CAD build for the part. Positions are in the model's coordinates, mm. Face numbers are marked on the shaded views. A direction names the side the tool comes from. Give positions to 0.01 mm unless a question says otherwise; leave off trailing zeros. Write each loop counter-clockwise with the first axis right and the second up, starting at its lowest first coordinate (ties: lowest second). Pieces come first, ordered by that corner, then holes. Notation, with made-up numbers: (-40, 5) - (-11, 5) arc R14 ccw to (-11, 21) - close; hole circle Ø7 at (32.25, -4). An arc over 180 degrees is marked (long way). Answer as a JSON object with one key per item and string values.
Solid Edge part; units mm, degrees
sketch "Sketch1" plane through (0, 0, 0) normal (0, -1, 0) x (1, 0, 0)
  line L0 (-8.05, -17.5) -> (8.05, -17.5)
  line L1 (8.05, -17.5) -> (8.05, 17.5)
  line L2 (8.05, 17.5) -> (-8.05, 17.5)
  line L3 (-8.05, 17.5) -> (-8.05, -17.5)
  dimension "D1" = 8.05
  dimension "D2" = 8.05
extrude "Protrusion1" add sketch "Sketch1" against normal blind 2
sketch "Sketch2" plane through (0, 0, 0) normal (0, -1, 0) x (1, 0, 0)
  line L0 (-10.05, -19.5) -> (10.05, -19.5)
  line L1 (10.05, -19.5) -> (10.05, 19.5)
  line L2 (10.05, 19.5) -> (-10.05, 19.5)
  line L3 (-10.05, 19.5) -> (-10.05, -19.5)
  line L4 (-8.05, -17.5) -> (8.05, -17.5)
  line L5 (8.05, -17.5) -> (8.05, 17.5)
  line L6 (8.05, 17.5) -> (-8.05, 17.5)
  line L7 (-8.05, 17.5) -> (-8.05, -17.5)
extrude "Extrusionsausprägung_2" add sketch "Sketch2" against normal blind 9
sketch "Sketch3" plane through (0, 0, 0) normal (0, -1, 0) x (1, 0, 0)
  circle A0 centre (0, 9.5) radius 5
extrude "Cutout1" cut sketch "Sketch3" against normal through all
sketch "Sketch4" plane through (0, 0, 0) normal (0, -1, 0) x (1, 0, 0)
  line L0 (-4.75, 7.9388) -> (4.75, 7.9388)
  line L1 (4.75, 7.9388) -> (4.75, -0.0612)
  line L2 (4.75, -0.0612) -> (-4.75, -0.0612)
  line L3 (-4.75, -0.0612) -> (-4.75, 7.9388)
  dimension "D1" = 4.75
  dimension "D2" = 4.75
extrude "Cutout2" cut sketch "Sketch4" against normal through all
chamfer "Fase_1" distance 0.5 angle 45 8 edges at (0, 9, 19.5) (0, 9, 17.5) (10.05, 9, 0) (8.05, 9, 0) (-8.05, 9, 0) (-10.05, 9, 0) (0, 9, -19.5) (0, 9, -17.5)
sketch "Sketch5" plane through (10.05, 5.75, 0) normal (1, 0, 0) x (0, 0, -1)
  line L0 (-19.5, -3.75) -> (-9.5, -3.75)
  line L1 (-9.5, -3.75) -> (-9.5, 3.25)
  line L2 (-9.5, 3.25) -> (-19.5, 3.25)
  line L3 (-19.5, 3.25) -> (-19.5, -3.75)
  line L4 (19.5, -3.75) -> (4.5, -3.75)
  line L5 (4.5, -3.75) -> (4.5, 3.25)
  line L6 (4.5, 3.25) -> (19.5, 3.25)
  line L7 (19.5, 3.25) -> (19.5, -3.75)
  dimension "D1" = 9.5
extrude "Cutout3" cut sketch "Sketch5" against normal through all
chamfer "Fase_3" distance 0.5 angle 45 8 edges at (10.05, 5.25, -4.5) (8.05, 5.25, -4.5) (-8.05, 5.25, -4.5) (-10.05, 5.25, -4.5) (-8.05, 5.25, 9.5) (-10.05, 5.25, 9.5) (8.05, 5.25, 9.5) (10.05, 5.25, 9.5)
sketch "Sketch6" plane through (0, 2, 0) normal (0, 1, 0) x (-1, 0, 0)
  line L0 (-10.05, 19.5) -> (10.05, 19.5)
  line L1 (10.05, 19.5) -> (10.05, 16.5)
  line L2 (10.05, 16.5) -> (-10.05, 16.5)
  line L3 (-10.05, 16.5) -> (-10.05, 19.5)
  dimension "D1" = 10.05
extrude "Cutout4" cut sketch "Sketch6" against normal through all
fillet "Verrundung_4" radius 7 2 edges at (10.05, 1, 16.5) (-10.05, 1, 16.5)
sketch "Sketch7" plane through (10.05, 4.25, -5) normal (1, 0, 0) x (0, -1, 0)
  line L0 (2.25, 14.5) -> (4.25, 14.5)
  line L1 (4.25, 14.5) -> (4.25, 3.5)
  line L2 (4.25, 3.5) -> (2.25, 3.5)
  line L3 (2.25, 3.5) -> (2.25, 14.5)
extrude "Cutout5" cut sketch "Sketch7" against normal through all
sketch "Sketch8" plane through (10.05, 4.25, 0.5) normal (1, 0, 0) x (0, -1, 0)
  arc A0 (2.25, 9) -> (-7.75, 19) centre (-7.75, 9) ccw
  line L0 (-7.75, 19) -> (-7.75, 21)
  arc A1 (-7.75, 21) -> (4.25, 9) centre (-7.75, 9) cw
  line L1 (4.25, 9) -> (2.25, 9)
extrude "Protrusion2" add sketch "Sketch8" against normal up to vertex (20.1 mm away)
fillet "Verrundung_5" radius 5 2 edges at (10.05, 12, -19.5) (-10.05, 12, -19.5)
fillet "Verrundung_6" radius 1.5 10 edges at (10.05, 1.9005, -14.9807) (10.05, 0, 0.5) (7.9997, 0, 14.4497) (0, 0, 16.5) (-7.9997, 0, 14.4497) (-10.05, 0, 0.5) (-10.05, 1.9005, -14.9807) (-8.6361, 10.4842, -20.4039) (0, 12, -20.5) (8.6361, 10.4842, -20.4039)
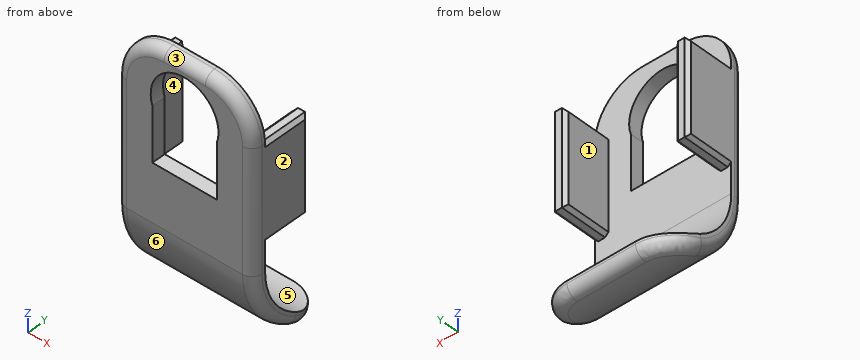
(1) Flat gauge pins, fed straight in: P1, Ø11.5, axis at x = 0, z = 9.5, coming from the +Y side; P2, Ø0.5, axis at x = 9, y = 5.5, coming from the +Z side; P3, Ø3, axis at x = -7, y = 1.5, coming from the +Z side. Where does each tip first touch, or does it go through?
Answer key:
{"P1": "stops at y = 2", "P2": "stops at z = 9.5", "P3": "stops at z = 16.06"}
(2) Saw through at A-A, the plane z = 7.5. Give the cut face in (x, y), and give its area (3 significant figures).
Answer key:
{"outline": "(-10.05, 1.5) arc R1.5 ccw to (-8.55, 0) - (-4.75, 0) - (-4.75, 2) - (-8.05, 2) - (-8.05, 8.5) - (-8.55, 9) - (-9.55, 9) - (-10.05, 8.5) - close; (4.75, 0) - (8.55, 0) arc R1.5 ccw to (10.05, 1.5) - (10.05, 8.5) - (9.55, 9) - (8.55, 9) - (8.05, 8.5) - (8.05, 2) - (4.75, 2) - close", "area": "47.7 mm²"}
(3) Saw through at B-B, the plane x = 0. Give the cut face in (y, z).
Answer key:
{"outline": "(0, -8.5) arc R12 ccw to (10.29, -20.38) arc R1.5 ccw to (12, -18.89) - (12, -18.5) arc R10 cw to (2, -8.5) - (2, -0.06) - (0, -0.06) - close; (0, 14.5) - (2, 14.5) - (2, 16.5) - (1.5, 16.5) arc R1.5 ccw to (0, 15) - close"}
(4) Saw through at C-C, the plane y = 4. State how many separate pieces and enclosed holes the cut face has, and give its area (3 significant figures).
Answer key:
{"separate pieces": "3", "enclosed holes": "0", "area": "113 mm²"}
(5) 3-axis set-ups, long thin cutter, end or side, ignore diameter. For the marked faces 4, 5 and 6: which of +Z, -Z, +X, -X, +Y, -Y reach the whole face in a straight line?
Answer key:
{"face 4": "+Z, +Y", "face 5": "+X, -X, +Y", "face 6": "-Z, +X, -X, -Y"}
(6) Probe L1, parallel to X at y = 8, z = 1; L2, parallel to Y at x = 3, z = -2; L3, parallel to Z at x = 0, y = 1.15. List the from-to ranges inside material, lowest first. Write a range as [from, to].
Answer key:
{"L1": "x = [-10.05, -8.05], [8.05, 10.05]", "L2": "y = [0, 2]", "L3": "z = [-13.63, -0.06], [14.5, 16.46]"}
(7) Pull direction X, two halves, no side cores. Call the marked faces 1, 2 and 3: pulls with the +X half, pulls with the -X half, needs draft (parallel to the pull), parting line crosses it, or undercut.
Answer key:
{"face 1": "undercut", "face 2": "pulls with the +X half", "face 3": "needs draft"}
